from build123d import *

# Parameters (mm, degrees)
F1_DEPTH       = 6
F3_DEPTH       = 25
F4_W           = 20
F4_H           = 30
F4_R           = 5
F5_DEPTH       = 5
F5_DEPTH_BACK  = 5
F10_W          = 30
F10_H          = 20
F10_R          = 5
F11_DEPTH      = 5
F11_DEPTH_BACK = 5
F16_W          = 30
F16_H          = 20
F16_R          = 5
F17_DEPTH      = 5
F17_DEPTH_BACK = 5


with BuildPart() as f1:
    # F0 (on Front) → F1 (new body)
    with BuildSketch(Plane.XZ):
        Polygon((28.612, 205.4420103874), (-28.612, 205.4420103874), (-118.612, 49.5574377062), (-90, 0), (90, 0), (118.612, 49.5574377062), align=None)
    extrude(amount=-F1_DEPTH)

    # F2 (on Front) → F3 (cut)
    with BuildSketch(Plane.XZ):
        Polygon((47.4997490062, 132.5), (-47.5002509938, 132.5), (-47.5002509938, 95), (-62.5002509938, 95), (-62.5002509938, 75), (-47.5002509938, 75), (-47.5002509938, 37.5), (47.4997490062, 37.5), (47.4997490062, 75), (62.4997490062, 75), (62.4997490062, 95), (47.4997490062, 95), align=None)
    extrude(amount=-F3_DEPTH, mode=Mode.SUBTRACT)

    # F4 (on Right) → F5 (join, two sides)
    with BuildSketch(Plane.YZ) as f5_sk:
        with Locations((16, 190.4420103874)):
            Rectangle(F4_W, F4_H)
        with Locations((16, 190.4420103874)):
            Circle(F4_R, mode=Mode.SUBTRACT)
    extrude(amount=F5_DEPTH)
    extrude(f5_sk.sketch, amount=-F5_DEPTH_BACK)

    # F10 (on 3pt) → F11 (join, two sides)
    with BuildSketch(Plane(origin=(36.806, 0, 63.7498620234), x_dir=(0.8660254038, 0, -0.5), z_dir=(0.5, 0, 0.8660254038))) as f11_sk:
        with Locations((62.9422863406, 16)):
            Rectangle(F10_W, F10_H)
        with Locations((62.9422863406, 16)):
            Circle(F10_R, mode=Mode.SUBTRACT)
    extrude(amount=F11_DEPTH)
    extrude(f11_sk.sketch, amount=-F11_DEPTH_BACK)

    # F16 (on 3pt) → F17 (join, two sides)
    with BuildSketch(Plane(origin=(-36.806, 0, 63.7498620234), x_dir=(0.8660254038, 0, 0.5), z_dir=(0.5, 0, -0.8660254038))) as f17_sk:
        with Locations((-62.9422863406, -16)):
            Rectangle(F16_W, F16_H)
        with Locations((-62.9422863406, -16)):
            Circle(F16_R, mode=Mode.SUBTRACT)
    extrude(amount=F17_DEPTH)
    extrude(f17_sk.sketch, amount=-F17_DEPTH_BACK)


solid = f1.part
Read the model definition and answer for the solid it produces. Units are mm, in the model's axes. A direction names the side the tool comes from. Coordinates: 2 decimals unless noted, no trailing zeros. Loops run counter-clockwise (first coordinate to the right, second up) from the corner with the lowest first, then second, coordinate; pieces in that order, holes last.
Q1. The part is cut by section A-A on z = 102. Write down the section's boundary in (x, y), and give its area (3 significant figures).
Q2. The part is cut by section B-B on y = 16. Write down the section's boundary in (x, z).
Q3. Which of the six approach directions +Z, -Z, +X, -X, +Y, -Y give full straight-line access (tool end or side, diameter ignored) to faces 5 (the face through (0, 16, 175.442)), 6 (the face through (-78.29, 16.14, 39.72)), 7 (the face through (-55, 3, 95)), 8 (the face through (-2, 6, 36)), 9 (the face through (-96.88, 20.3, 34.84))?
Q4. The mould has two halves that part along Z. Classify faces 1 (the face through (0, 6, 205.442)), 2 (the face through (-91.88, 20.3, 26.18)), 3 (the face through (-5, 20, 194)), 4 (the face through (-62.5, 3, 85)): +Z half, -Z half, draft (parallel to the pull), parting line (faces both ways), or undercut.
Q5. Consider probe 1 along Z at (x, y) = (-1.75, 16); probe 2 along Y at (x, z) = (-95.5, 49.5); probe 3 along X at (y, z) = (18.5, 178.5). Determine where each line is inside the solid, lowest interval first.
Q6. The part is cut by section D-D on z = 168. Write down the section's boundary in (x, y).
Q7. Each of these flat-tipped pins is pushed along its axis until it touches: pin 1 Ø3 at (x, y) = (-54, 4) entering from -Z; pin 2 Ø1 at (x, y) = (-94.5, 22.5) entering from -Z; pin 3 Ø11.5 at (y, z) = (16, 190.44) entering from +X; pin 4 Ø5 at (y, z) = (3.5, 84) entering from -X. Where does it stop, or does it pass through?
Q8. The part is cut by section C-C on x = 58. Write down the section's boundary in (y, z).
Results below:
1. outline: (-88.33, 0) - (-47.5, 0) - (-47.5, 6) - (-88.33, 6) - close; (47.5, 0) - (88.33, 0) - (88.33, 6) - (47.5, 6) - close
1. area: 490 mm2
2. outline: (-106.81, 29.11) - (-101.81, 20.45) - (-93.15, 25.45) - (-98.15, 34.11) - close; (-89.49, 39.11) - (-84.49, 30.45) - (-75.83, 35.45) - (-80.83, 44.11) - close; (-5, 175.44) - (5, 175.44) - (5, 185.44) - (-5, 185.44) - close; (-5, 195.44) - (5, 195.44) - (5, 205.44) - (-5, 205.44) - close; (75.83, 35.45) - (84.49, 30.45) - (89.49, 39.11) - (80.83, 44.11) - close; (93.15, 25.45) - (101.81, 20.45) - (106.81, 29.11) - (98.15, 34.11) - close
3. face 5: -Z, +X, -X, +Y
3. face 6: +Z, +Y
3. face 7: +Y, -Y
3. face 8: +Y
3. face 9: +Z, -X, +Y
4. face 1: +Z half
4. face 2: -Z half
4. face 3: draft
4. face 4: undercut
5. probe 1: z = 175.44 to 185.44, 195.44 to 205.44
5. probe 2: y = 0 to 6
5. probe 3: x = -5 to 5
6. outline: (-50.23, 0) - (50.23, 0) - (50.23, 6) - (-50.23, 6) - close
7. pin 1: stops at z = 0
7. pin 2: stops at z = 24.38
7. pin 3: stops at x = 5
7. pin 4: stops at x = -100.17
8. outline: (0, 0) - (6, 0) - (6, 75) - (0, 75) - close; (0, 95) - (6, 95) - (6, 154.54) - (0, 154.54) - close
